```python
from build123d import *

# Parameters (mm, degrees)
SKETCH_1_W          = 70
SKETCH_1_H          = 74
EXTRUDE_1_DEPTH     = 5
CUT_EXTRUDE_2_REACH = 103.985
SKETCH_2_W          = 60
SKETCH_2_H          = 2.5
SKETCH_3_W          = 56.4
SKETCH_3_H          = 56.4
CUT_EXTRUDE_3_DEPTH = 20
SKETCH_4_W          = 3.6
SKETCH_4_H          = 61.4
CUT_EXTRUDE_5_DEPTH = 102.985293057


with BuildPart() as part:
    # Эскиз1 → Вытянуть1 (new body)
    with BuildSketch(Plane.XY):
        with Locations((35, 37)):
            Rectangle(SKETCH_1_W, SKETCH_1_H)
    extrude(amount=EXTRUDE_1_DEPTH)

    # Эскиз2 → Вытянуть2 (cut, up to next)
    with BuildSketch(Plane.XY.offset(5), mode=Mode.PRIVATE) as cut_extrude_2_sk1:
        with Locations((35, 6.25)):
            Rectangle(SKETCH_2_W, SKETCH_2_H)
    cut_extrude_2_tool1 = extrude(cut_extrude_2_sk1.sketch, amount=-CUT_EXTRUDE_2_REACH, mode=Mode.PRIVATE) & part.part
    add(cut_extrude_2_tool1.solids().sort_by_distance((35, 6.25, 5))[0], mode=Mode.SUBTRACT)

    # Эскиз3 → Вытянуть3 (cut)
    with BuildSketch(Plane.XY.offset(5)):
        with Locations((33.2, 40.8)):
            Rectangle(SKETCH_3_W, SKETCH_3_H)
    extrude(amount=-CUT_EXTRUDE_3_DEPTH, mode=Mode.SUBTRACT)

    # Эскиз4 → Вытянуть5 (cut, through all)
    with BuildSketch(Plane(origin=(0, 0, 0), x_dir=(-1, 0, 0), z_dir=(0, 0, -1))):
        with Locations((-68.2, 43.3)):
            Rectangle(SKETCH_4_W, SKETCH_4_H)
    extrude(amount=-CUT_EXTRUDE_5_DEPTH, mode=Mode.SUBTRACT)


solid = part.part
```
The model under review builds one solid part; all positions refer to its coordinate system, in mm. A direction names the side the tool comes from. Give positions to 0.01 mm unless a question says otherwise; leave off trailing zeros. Write each loop counter-clockwise with the first axis right and the second up, starting at its lowest first coordinate (ties: lowest second). Pieces come first, ordered by that corner, then holes. Notation, with made-up numbers: (54.5, 52.5) - (112.5, 52.5) arc R20 cw to (112.5, 80.5) - close; hole circle Ø6 at (31.25, 77.25). An arc over 180 degrees is marked (long way). Answer in a Markdown table with one row per item. Add a question column.
1. We need section B-B on x = 27. Write out the cut boundary in (y, z).
2. We need section A-A on y = 56. Write out the cut boundary in (x, z), then the cut area to 3 significant figures.
3. Draft analysis for pull direction Y (two halves, no side actions). For faces 4 (the flat face through (3, 38, 5)), 5 (the flat face through (68, 12.6, 2)), 6 (the flat face through (33, 12.6, 3)), state which applies: +Y half, -Y half, draft (parallel to the pull), parting line (faces both ways), or undercut.
4. Tool access review of faces 1 (the flat face through (66.4, 43, 2)), 2 (the flat face through (0, 36, 2)), 3 (the flat face through (35, 7.5, 3)): name each direction out of +Z, -Z, +X, -X, +Y, -Y from which nothing blocks a thin tool from reaching the whole face with its end or side.
5. Insertion check: P1, Ø1.8, axis at x = 69, z = 1.5, coming from the +Y side; P2, Ø1.5, axis at y = 20, z = 2, coming from the +X side. Each pin has a flat end and moves straight along its axis. Give the tip position at first contact, or say it passes through.
6. We need section C-C on z = 2.5. Write out the cut boundary in (x, y).
7. Wall thickness on line 1 along Y through (x, z) = (17, 3.9); line 2 along X through (y, z) = (59.5, 0.3); line 3 along Y through (x, z) = (64.5, 0.95): over which ranges is each line inside the solid? List them lowest first. Write a range as [from, to].
Ans:
| question | item | result |
|---|---|---|
| 1 | outline | (0, 0) - (5, 0) - (5, 5) - (0, 5) - close; (7.5, 0) - (12.6, 0) - (12.6, 5) - (7.5, 5) - close; (69, 0) - (74, 0) - (74, 5) - (69, 5) - close |
| 2 | outline | (0, 0) - (5, 0) - (5, 5) - (0, 5) - close; (61.4, 0) - (66.4, 0) - (66.4, 5) - (61.4, 5) - close |
| 2 | area | 50.0 mm^2 |
| 3 | face 4 | draft |
| 3 | face 5 | +Y half |
| 3 | face 6 | undercut |
| 4 | face 1 | +Z, -Z, +X, +Y |
| 4 | face 2 | +Z, -Z, -X, +Y, -Y |
| 4 | face 3 | +Z, -Z |
| 5 | P1 | stops at y = 12.6 |
| 5 | P2 | stops at x = 66.4 |
| 6 | outline | (0, 0) - (70, 0) - (70, 12.6) - (66.4, 12.6) - (66.4, 74) - (0, 74) - close; hole (5, 5) - (65, 5) - (65, 7.5) - (5, 7.5) - close; hole (5, 12.6) - (61.4, 12.6) - (61.4, 69) - (5, 69) - close |
| 7 | line 1 | y = [0, 5], [7.5, 12.6], [69, 74] |
| 7 | line 2 | x = [0, 5], [61.4, 66.4] |
| 7 | line 3 | y = [0, 5], [7.5, 74] |
